from build123d import *

# Parameters (mm, degrees)
F1_DEPTH      = 76.2
F1_DEPTH_BACK = 76.2
F3_DEPTH      = 6.35
F3_DEPTH_BACK = 6.35


with BuildPart() as f1:
    # F0 (on Right) → F1 (new body, two sides)
    with BuildSketch(Plane.YZ) as f1_sk:
        Polygon((-10.471897, -31.062707), (33.533607, 26.356237), (24.355987, 26.826883), (-12.354486, -20.237826), (-27.415192, -20.237826), (-21.767426, -6.589059), (-29.768426, -6.589059), (-42.005252, -31.062707), align=None)
    extrude(amount=F1_DEPTH)
    extrude(f1_sk.sketch, amount=-F1_DEPTH_BACK)

    # F2 (on Right) → F3 (join, two sides)
    with BuildSketch(Plane.YZ) as f3_sk:
        Polygon((38.475402, -35.063207), (22.944046, 16.943295), (15.649015, 8.001001), (28.59181, -35.063207), align=None)
    extrude(amount=F3_DEPTH)
    extrude(f3_sk.sketch, amount=-F3_DEPTH_BACK)


solid = f1.part
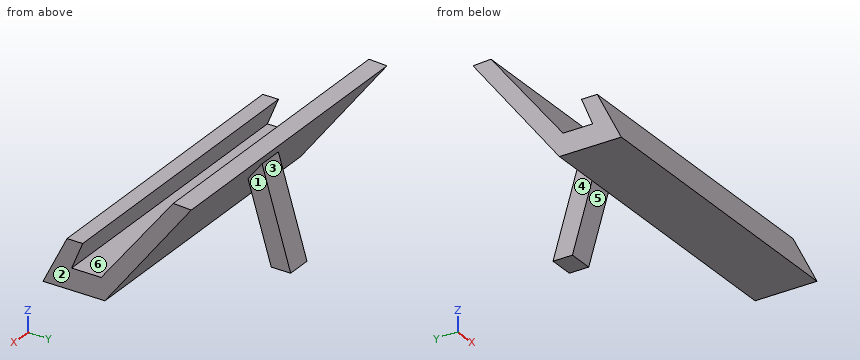
Geometry check sheet. Reference: the model listing, model coordinates, mm. Face numbers are marked on the shaded views. A direction names the side the tool comes from. Give positions to 0.01 mm unless a question says otherwise; leave off trailing zeros. Order: outer loops, then holes, each group sorted by start corner. A loop starts at its lowest first (then second) coordinate and runs counter-clockwise, first axis right, second up. Notation, with made-up numbers: M 31,30 L 65,30 A35 cw 65,64 Z; hole C -17.5,-10 d10. An arc over 180 degrees is marked long. Use a Markdown table: item, result.
Item 1: Depth check by flat-ended pin: P1, Ø4, axis at x = -42, z = -1, coming from the -Y side; P2, Ø17.5, axis at y = 24, z = -19.5, coming from the +X side; P3, Ø1.5, axis at x = -10.5, z = 19.5, coming from the +Y side. Enter the tip coordinate at first touch or a pass-through.
Answers follow:
| item | result |
|---|---|
| P1 | stops at y = 1.09 |
| P2 | stops at x = 6.35 |
| P3 | stops at y = 28.85 |
Item 2: Material ranges on line 1 along Z through (x, y) = (-43.5, -17); line 2 along Y through (x, z) = (61.5, -8); line 3 along Y through (x, z) = (-26.5, -9), recorded low to high.
Answers follow:
| item | result |
|---|---|
| line 1 | z = -31.06 to -20.24 |
| line 2 | y = -30.47 to -22.35, -2.81 to 7.2 |
| line 3 | y = -30.97 to -22.77, -3.59 to 6.44 |
Item 3: Section check B-B (x = 12). Record the cut outline in (y, z), and give its area (3 significant figures).
Answers follow:
| item | result |
|---|---|
| outline | M -42.01,-31.06 L -10.47,-31.06 L 33.53,26.36 L 24.36,26.83 L -12.35,-20.24 L -27.42,-20.24 L -21.77,-6.59 L -29.77,-6.59 Z |
| area | 936 mm2 |
Item 4: Tool access check on the marked faces 1 and 2. Record the directions out of +Z, -Z, +X, -X, +Y, -Y that give a thin tool (end or side, any length) a straight path to the whole face; none if there is none.
Answers follow:
| item | result |
|---|---|
| face 1 | -Z, +X, +Y |
| face 2 | +Z, -Z, +X, +Y, -Y |
Item 5: Section check D-D (y = 13.5). Record the cut outline in (x, z), and give its area (3 significant figures).
Answers follow:
| item | result |
|---|---|
| outline | M -76.2,0.22 L 76.2,0.22 L 76.2,12.91 L -76.2,12.91 Z |
| area | 1,930 mm2 |
Item 6: Section check C-C (z = 11). Record the cut outline in (x, y), and give its area (3 significant figures).
Answers follow:
| item | result |
|---|---|
| outline | M -76.2,12.01 L 76.2,12.01 L 76.2,21.76 L 6.35,21.76 L 6.35,24.72 L -6.35,24.72 L -6.35,21.76 L -76.2,21.76 Z |
| area | 1,520 mm2 |
Item 7: Draft check along Y on the marked faces 3, 4, 5 and 6. Enter one of: +Y half, -Y half, draft (parallel to the pull), parting line (faces both ways), or undercut.
Answers follow:
| item | result |
|---|---|
| face 3 | +Y half |
| face 4 | draft |
| face 5 | undercut |
| face 6 | undercut |
Item 8: Section check A-A (z = 1.5). Record the cut outline in (x, y), and give its area (3 significant figures).
Answers follow:
| item | result |
|---|---|
| outline | M -76.2,4.6 L 76.2,4.6 L 76.2,14.48 L -76.2,14.48 Z; M -6.35,17.6 L 6.35,17.6 L 6.35,27.56 L -6.35,27.56 Z |
| area | 1,630 mm2 |
